```python
from build123d import *

# Parameters (mm, degrees)
F3_DEPTH = 6.35
F5_DEPTH = 25.4
F7_DEPTH = 3.175


with BuildPart() as f1:
    # F0 (on Front) → F1 (revolve)
    with BuildSketch(Plane.XZ):
        Polygon((59.4741, 0), (0, 0), (0, -12.7508), (50.8, -12.7508), (50.8, -5.626218), (59.4741, -3.302), align=None)
    revolve(axis=Axis((0, 0, -6.3754), (0, 0, -1)))

    # F2 (on face) → F3 (cut)
    with BuildSketch(Plane.XY):
        with BuildLine():
            Line((-40.64, -4.826), (-38.1, -4.826))
            ThreePointArc((-38.1, -4.826), (-33.274, 0), (-38.1, 4.826))
            Line((-38.1, 4.826), (-40.64, 4.826))
            ThreePointArc((-40.64, 4.826), (-45.466, 0), (-40.64, -4.826))
        make_face()
    extrude(amount=-F3_DEPTH, mode=Mode.SUBTRACT)

    # F4 (on face) → F5 (cut)
    with BuildSketch(Plane.XY):
        with BuildLine():
            ThreePointArc((-59.346964, -0.127), (-59.3471, 0), (-59.346964, 0.127))
            Line((-59.346964, 0.127), (-59.4741, 0.127))
            Line((-59.4741, 0.127), (-59.4741, -0.127))
            Line((-59.4741, -0.127), (-59.346964, -0.127))
        make_face()
    extrude(amount=-F5_DEPTH, mode=Mode.SUBTRACT)

    # F6 (on face) → F7 (cut)
    with BuildSketch(Plane(origin=(0, 0, -12.7508), x_dir=(1, 0, 0), z_dir=(0, 0, -1))):
        Polygon((3.175, -25.4), (3.175, 0), (3.175, 25.4), (-3.175, 25.4), (-3.175, 0), (-3.175, -25.4), align=None)
    extrude(amount=-F7_DEPTH, mode=Mode.SUBTRACT)


solid = f1.part
```
The listing builds one solid part. Answer for the finished solid, in the listing's coordinates (mm). A direction names the side the tool comes from. Coordinates: 2 decimals unless noted, no trailing zeros. Loops run counter-clockwise (first coordinate to the right, second up) from the corner with the lowest first, then second, coordinate; pieces in that order, holes last. Notation, with made-up numbers: (28.25, 71.5) -> (40.25, 71.5) arc R32 ccw to (40.25, 100.5) -> close; hole circle Ø1 at (52, -28.5). An arc over 180 degrees is marked (long way). Return JSON: item names as keys, results as strings. Group by question number.
(1) Given pin 1 Ø0.8 at (x, z) = (-39.5, -2) entering from -Y; pin 2 Ø4 at (x, y) = (-26, -46.5) entering from -Z; pin 3 Ø3 at (x, y) = (-39, 0.5) entering from +Z; pin 4 Ø2 at (x, y) = (-45.5, 40) entering from +Z, each flat-ended and moving along its own axis, determine where each tip first touches the part or whether it passes through.
(2) A cutting plane is placed at A-A on x = 0. Write down the section's boundary in (y, z), and give its area (3 significant figures).
(3) Which of the six approach directions +Z, -Z, +X, -X, +Y, -Y give full straight-line access (tool end or side, diameter ignored) to faces 4 (the flat face through (-11, -1, -12.751)), 5 (the flat face through (-39, 0, -6.35)), 6 (the flat face through (-3.175, 0, -11))?
(4) Determine the mould class of faces 1 (the flat face through (-1, -1, 0)), 2 (the cylindrical face through (-11.012, 49.592, -9.139)), 3 (the flat face through (0, 0, -9.576)) for opening direction X: released by +X, released by -X, zero draft, split by the parting line, or undercut.
(5) Find the intervals of material crossed by probe 1 along Y at (x, z) = (1, -8); probe 2 along Y at (x, z) = (1.5, -2.5); probe 3 along Y at (x, z) = (-40, -1), in increasing order. Write a range as from..to.
The answers:
{
 "1": {"pin 1": "stops at y = -44.81", "pin 2": "stops at z = -5.5", "pin 3": "stops at z = -6.35", "pin 4": "passes through"},
 "2": {"outline": "(-59.47, -3.3) -> (-50.8, -5.63) -> (-50.8, -12.75) -> (-25.4, -12.75) -> (-25.4, -9.58) -> (25.4, -9.58) -> (25.4, -12.75) -> (50.8, -12.75) -> (50.8, -5.63) -> (59.47, -3.3) -> (59.47, 0) -> (-59.47, 0) -> close", "area": "1,210 mm^2"},
 "3": {"face 4": "-Z, +X, -X, +Y, -Y", "face 5": "+Z", "face 6": "-Z"},
 "4": {"face 1": "zero draft", "face 2": "split by the parting line", "face 3": "undercut"},
 "5": {"probe 1": "y = -50.79..50.79", "probe 2": "y = -59.46..59.46", "probe 3": "y = -44.01..-4.83, 4.83..44.01"}
}
